Model file for the job. Use its own axes, mm. A direction names the side the tool comes from. Give positions to 0.01 mm unless a question says otherwise; leave off trailing zeros. Write each loop counter-clockwise with the first axis right and the second up, starting at its lowest first coordinate (ties: lowest second). Pieces come first, ordered by that corner, then holes.
```python
from build123d import *

# Parameters (mm, degrees)
SKETCH_W    = 80
SKETCH_H    = 122.16
SKETCH_R    = 2
SKETCH_W_2  = 60
SKETCH_H_2  = 102.16
PAD_DEPTH   = 10
FILLET_R    = 1
FILLET001_R = 1


with BuildPart() as part:
    # Sketch → Pad (new body)
    with BuildSketch(Plane.XY):
        with Locations((45, 66.08)):
            Rectangle(SKETCH_W, SKETCH_H)
        with Locations((10, 99.16)):
            Circle(SKETCH_R, mode=Mode.SUBTRACT)
        with Locations((10, 33)):
            Circle(SKETCH_R, mode=Mode.SUBTRACT)
        with Locations((80, 99.16)):
            Circle(SKETCH_R, mode=Mode.SUBTRACT)
        with Locations((80, 33)):
            Circle(SKETCH_R, mode=Mode.SUBTRACT)
        with Locations((45, 122.16)):
            Circle(SKETCH_R, mode=Mode.SUBTRACT)
        with Locations((45, 10)):
            Circle(SKETCH_R, mode=Mode.SUBTRACT)
        with Locations((45, 66.08)):
            Rectangle(SKETCH_W_2, SKETCH_H_2, mode=Mode.SUBTRACT)
    extrude(amount=PAD_DEPTH)

    # Fillet
    fillet_edges = [part.edges().sort_by_distance(p)[0] for p in [
        (45, 117.16, 10),
        (15, 66.08, 10),
    ]]
    fillet(fillet_edges, radius=FILLET_R)

    # Fillet001
    fillet001_edges = [part.edges().sort_by_distance(p)[0] for p in [
        (45, 15, 10),
        (75, 66.08, 10),
    ]]
    fillet(fillet001_edges, radius=FILLET001_R)


solid = part.part
```
1. Pull direction Y, two halves, no side cores. Call faces 3 (the flat face through (45, 15, 4)), 4 (the flat face through (85, 65, 5)), 5 (the flat face through (44, 5, 5)): +Y half, -Y half, draft (parallel to the pull), parting line (faces both ways), or undercut.
Calculated:
face 3: undercut
face 4: draft
face 5: -Y half
2. Which spindle directions (+Z, -Z, +X, -X, +Y, -Y) get a long thin tool onto all of the face, cutting with end or side? Do faces 1 (the flat face through (45, 117.16, 4)), 2 (the flat face through (9, 67, 10)). Say none if no direction does.
Calculated:
face 1: +Z, -Z
face 2: +Z, +X, -X, +Y, -Y
3. Pin check, flat tips, straight feed: P1, Ø3.5, axis at x = 45, y = 10, coming from the -Z side; P2, Ø6.5, axis at x = 45, y = 122.16, coming from the -Z side. Stop position of each tip, or through.
Calculated:
P1: passes through
P2: stops at z = 0
4. Probe probe 1 along Y at (x, z) = (80, 2.5); probe 2 along Y at (x, z) = (59.5, 4.5); probe 3 along X at (y, z) = (108, 6). List the from-to ranges inside material, lowest first.
Calculated:
probe 1: y = 5 to 31, 35 to 97.16, 101.16 to 127.16
probe 2: y = 5 to 15, 117.16 to 127.16
probe 3: x = 5 to 15, 75 to 85
5. Slice it at B-B, the plane x = 45. Write the cut outline in (y, z), and give its area (3 significant figures).
Calculated:
outline: (5, 0) - (8, 0) - (8, 10) - (5, 10) - close; (12, 0) - (15, 0) - (15, 9) arc R1 ccw to (14, 10) - (12, 10) - close; (117.16, 0) - (120.16, 0) - (120.16, 10) - (118.16, 10) arc R1 ccw to (117.16, 9) - close; (124.16, 0) - (127.16, 0) - (127.16, 10) - (124.16, 10) - close
area: 120 mm2
6. Slice it at C-C, the plane y = 46. Write the cut outline in (x, z).
Calculated:
outline: (5, 0) - (15, 0) - (15, 9) arc R1 ccw to (14, 10) - (5, 10) - close; (75, 0) - (85, 0) - (85, 10) - (76, 10) arc R1 ccw to (75, 9) - close
7. Slice it at D-D, the plane x = 10. Write the cut outline in (y, z).
Calculated:
outline: (5, 0) - (31, 0) - (31, 10) - (5, 10) - close; (35, 0) - (97.16, 0) - (97.16, 10) - (35, 10) - close; (101.16, 0) - (127.16, 0) - (127.16, 10) - (101.16, 10) - close
8. Slice it at A-A, the plane y = 99.16. Write the cut outline in (x, z).
Calculated:
outline: (5, 0) - (8, 0) - (8, 10) - (5, 10) - close; (12, 0) - (15, 0) - (15, 9) arc R1 ccw to (14, 10) - (12, 10) - close; (75, 0) - (78, 0) - (78, 10) - (76, 10) arc R1 ccw to (75, 9) - close; (82, 0) - (85, 0) - (85, 10) - (82, 10) - close
